Build history of the part. All positions in model axes, mm. Round coordinates to 2 decimals unless told otherwise and drop trailing zeros. Write each loop counter-clockwise with the first axis right and the second up, starting at its lowest first coordinate (ties: lowest second). Pieces come first, ordered by that corner, then holes. Notation, with made-up numbers: M 74,77 L 127,77 A23 ccw 127,102 Z; hole C -31,-38.75 d3. An arc over 180 degrees is marked long. One line per item, written item: value. Start each with the question number.
```python
from build123d import *

# Parameters (mm, degrees)
F1_DEPTH = 19.05
F2_R     = 1.5875
F3_DEPTH = 6.351
F4_R     = 1.5875
F5_DEPTH = 19.051


with BuildPart() as f1:
    # F0 (on Front) → F1 (new body)
    with BuildSketch(Plane.XZ):
        Polygon((1.833087, 3.175), (-1.833087, 3.175), (-3.666174, 0), (-1.833087, -3.175), (1.833087, -3.175), (3.666174, 0), align=None)
    extrude(amount=F1_DEPTH)

    # F2 (on face) → F3 (cut, through all)
    with BuildSketch(Plane.XY.offset(3.175)):
        with Locations((0, -6.35)):
            Circle(F2_R)
    extrude(amount=-F3_DEPTH, mode=Mode.SUBTRACT)

    # F4 (on face) → F5 (cut, through all)
    with BuildSketch(Plane.XZ.offset(19.05)):
        Circle(F4_R)
    extrude(amount=-F5_DEPTH, mode=Mode.SUBTRACT)


solid = f1.part
```
Item 1: Cut at B-B, the plane y = -17. Write the cut outline in (x, z) (1 decimal).
Item 2: Drill centre lines: line 1 (Z direction, x = 0, y = -11.5) (1 decimal); line 2 (Y direction, x = -1, z = -2); line 3 (X direction, y = -6, z = 0.75). Where is each one in solid material? Low to high.
Item 3: Cut at A-A, the plane x = 0. Count the separate pieces of the cut face and the enclosed holes in it, plus the area to 3 significant figures.
Item 4: Drop a flat-ended pin along its axis: pin 1 (3 mm diameter, centred on x = -2, z = 0, fed in from +Y). Give the stop position or say it passes through.
Item 5: Two-plate mould, pull along Z, no slides. Class faces 1 (the flat face through (0, -9, 3.175)), 2 (the flat face through (2, -19.05, 1)), 3 (the cylindrical face through (1.514, -12.789, 0.477)): pulls with the +Z half, pulls with the -Z half, needs draft (parallel to the pull), parting line crosses it, or undercut.
Item 6: Cut at D-D, the plane y = -5.25. Write the cut outline in (x, z) (1 decimal).
Computed values:
1. outline: M -3.7,0 L -1.8,-3.2 L 1.8,-3.2 L 3.7,0 L 1.8,3.2 L -1.8,3.2 Z; hole C 0,0 d3.2
2. line 1: z = -3.2 to -1.6, 1.6 to 3.2
2. line 2: y = -19.05 to -7.58, -5.12 to 0
2. line 3: x = -3.23 to -1.55, 1.55 to 3.23
3. separate pieces: 4
3. enclosed holes: 0
3. area: 50.4 mm2
4. pin 1: stops at y = 0
5. face 1: pulls with the +Z half
5. face 2: needs draft
5. face 3: undercut
6. outline: M -3.7,0 L -1.8,-3.2 L -1.1,-3.2 L -1.1,-1.1 A1.6 cw -1.1,1.1 L -1.1,3.2 L -1.8,3.2 Z; M 1.1,-3.2 L 1.8,-3.2 L 3.7,0 L 1.8,3.2 L 1.1,3.2 L 1.1,1.1 A1.6 cw 1.1,-1.1 Z
